from build123d import *

# Parameters (mm, degrees)
SKETCH1_R          = 205.4
SKETCH1_R_2        = 185.4
BODY_DEPTH         = 5
SKETCH2_R          = 4
CUT_EXTRUDE1_DEPTH = 11
HOLES_COUNT        = 6


with BuildPart() as part:
    # Sketch1 → Body (new body, symmetric)
    with BuildSketch(Plane.XY):
        Circle(SKETCH1_R)
        Circle(SKETCH1_R_2, mode=Mode.SUBTRACT)
    extrude(amount=BODY_DEPTH, both=True)

    # Sketch2 → Cut-Extrude1 (cut, through all)
    with BuildSketch(Plane.XY.offset(5)):
        with Locations((0, 195.4)):
            Circle(SKETCH2_R)
    cut_extrude1 = extrude(amount=-CUT_EXTRUDE1_DEPTH, mode=Mode.SUBTRACT)

    # Holes: Cut-Extrude1 ×6 about axis
    holes_axis = Axis((0, 0, 0), (0, 0, 1))
    for i in range(1, HOLES_COUNT):
        add(cut_extrude1.rotate(holes_axis, i * 360 / HOLES_COUNT), mode=Mode.SUBTRACT)


solid = part.part
Geometry: final body of the model. Coordinates: model frame, mm. Give positions to 0.01 mm unless a question says otherwise; leave off trailing zeros. Loops run counter-clockwise (first coordinate to the right, second up) from the corner with the lowest first, then second, coordinate; pieces in that order, holes last. Notation, with made-up numbers: (-8.5, 44.25) - (22.5, 44.25) arc R18 ccw to (22.5, 66.25) - close; hole circle Ø7 at (53, 84). An arc over 180 degrees is marked (long way). One line per question, with ' | ' between items. Start each with the question number.
(1) Section query A-A on y = 0. Return loops of the section in (x, z), then the cut area to 3 significant figures.
(2) Section query B-B on x = 86. Return loops of the section in (y, z), then the cut area to 3 significant figures.
(3) Contact query for flat-ended pins moving along their axis: pin 1 (6.5 mm diameter, centred on x = -169.22, y = -97.7, fed in from +Z); pin 2 (3 mm diameter, centred on x = -109.5, z = 1, fed in from -Y); pin 3 (3 mm diameter, centred on x = 27, z = 3, fed in from -Y); pin 4 (1 mm diameter, centred on x = 114, z = 0, fed in from +Y). Output: stop coordinate, or through.
(4) Ray query, line 1 (Y direction, x = 0.5, z = -3.5); line 2 (X direction, y = 100.5, z = 3.75); line 3 (Y direction, x = -4.5, z = -1.25). Return the intervals inside material, ascending. Write a range as from..to.
(5) Section query C-C on z = -0.25. Return loops of the section in (x, y), then the cut area to 3 significant figures.
(6) Pull-direction query (Y, two-part tool) for faces 1 (the cylindrical face through (-147.13, -112.81, -0.07)), 2 (the flat face through (-153, -106, 5)), 3 (the cylindrical face through (-205.2, 9.03, 0.07)); classes: released by +Y, released by -Y, zero draft, split by the parting line, or undercut.
The answers:
1) outline: (-205.4, -5) - (-185.4, -5) - (-185.4, 5) - (-205.4, 5) - close; (185.4, -5) - (205.4, -5) - (205.4, 5) - (185.4, 5) - close | area: 400 mm2
2) outline: (-186.53, -5) - (-164.25, -5) - (-164.25, 5) - (-186.53, 5) - close; (164.25, -5) - (186.53, -5) - (186.53, 5) - (164.25, 5) - close | area: 446 mm2
3) pin 1: through | pin 2: y = -174.71 | pin 3: y = -203.81 | pin 4: y = 171.19
4) line 1: -205.4..-199.37, -191.43..-185.4, 185.4..191.43, 199.37..205.4 | line 2: -179.13..-172.08, -166.36..-155.8, 155.8..166.36, 172.08..179.13 | line 3: -205.35..-185.35, 185.35..205.35
5) outline: circle Ø410.8 at (0, 0); hole circle Ø370.8 at (0, 0); hole circle Ø8 at (-169.22, -97.7); hole circle Ø8 at (-169.22, 97.7); hole circle Ø8 at (0, -195.4); hole circle Ø8 at (0, 195.4); hole circle Ø8 at (169.22, -97.7); hole circle Ø8 at (169.22, 97.7) | area: 24,300 mm2
6) face 1: undercut | face 2: zero draft | face 3: split by the parting line
